```python
from build123d import *


with BuildPart() as part:
    # Croquis1 → Revolución1 (revolve)
    with BuildSketch(Plane.XY):
        Polygon((2.5, 199.2), (0, 199.2), (0, 0), (80, 0), (80, 176.605), (2.5, 176.605), align=None)
        Polygon((80, 0), (0, 0), (0, -199.2), (2.5, -199.2), (2.5, -176.605), (80, -176.605), align=None)
    revolve(axis=Axis((0, 415.25313391, 0), (0, -1, 0)))


solid = part.part
```
For this review, take the finished solid that the model builds, in its own axes (mm). Round coordinates to 2 decimals unless told otherwise and drop trailing zeros. Order: outer loops, then holes, each group sorted by start corner. A loop starts at its lowest first (then second) coordinate and runs counter-clockwise, first axis right, second up. Notation, with made-up numbers: (67.5, 8.25) -> (110.5, 8.25) arc R20 cw to (110.5, 24.25) -> close; hole circle Ø8 at (7, -13.75). An arc over 180 degrees is marked (long way). Use a Markdown table: item, result.
Item 1: Take a section at C-C (z = -17.5). State the section outline as (x, y) points (3 decimals), plus the area to 3 significant figures.
Resolved:
| item | result |
|---|---|
| outline | (-78.062, -176.605) -> (78.062, -176.605) -> (78.062, 176.605) -> (-78.062, 176.605) -> close |
| area | 55,100 mm² |
Item 2: Take a section at A-A (y = -68.5). State the section outline as (x, z) points.
Resolved:
| item | result |
|---|---|
| outline | circle Ø160 at (0, 0) |
Item 3: Take a section at B-B (x = 17.5). State the section outline as (y, z) points (3 decimals).
Resolved:
| item | result |
|---|---|
| outline | (-176.605, -78.062) -> (176.605, -78.062) -> (176.605, 78.062) -> (-176.605, 78.062) -> close |
Item 4: For line 1 along Y through (x, z) = (-57.5, -37.5) (3 decimals); line 2 along Z through (x, y) = (2, 147) (3 decimals); line 3 along X through (y, z) = (106, 68), list the stretches that pass through material, from the lowest coordinate up. Write a range as [from, to].
Resolved:
| item | result |
|---|---|
| line 1 | y = [-176.605, 176.605] |
| line 2 | z = [-79.975, 79.975] |
| line 3 | x = [-42.14, 42.14] |
Item 5: For pin 1 (8 mm diameter, centred on x = 22.5, z = 17, fed in from +Y) (3 decimals); pin 2 (2 mm diameter, centred on x = -48, y = 100.5, fed in from +Z); pin 3 (6 mm diameter, centred on y = 93.5, z = -31.5, fed in from -X), all flat-tipped, find the tip position at first contact; note any pin that passes through.
Resolved:
| item | result |
|---|---|
| pin 1 | stops at y = 176.605 |
| pin 2 | stops at z = 64.74 |
| pin 3 | stops at x = -74.75 |
